Here's how the part is built. I have some questions about the finished solid (model axes, mm). Face numbers are marked on the shaded views. Coordinates: 2 decimals unless noted, no trailing zeros. Loops run counter-clockwise (first coordinate to the right, second up) from the corner with the lowest first, then second, coordinate; pieces in that order, holes last. Notation, with made-up numbers: (8, -37) -> (21, -37) arc R14 ccw to (21, -28) -> close; hole circle Ø1 at (85, 22). An arc over 180 degrees is marked (long way). Answer as a JSON object with one key per item and string values. Group by question number.
1) I want a section at C-C (x = 80). Write out the boundary of the cut face in (y, z), then the cut area to 3 significant figures.
2) I need wall thicknesses on probe 1 along Y at (x, z) = (80, -1); probe 2 along Y at (x, z) = (130, 3); probe 3 along X at (y, z) = (54, 11.25). Which ranges of each line are inside material? Lowest first, please. Write a range as [from, to].
3) I want a section at B-B (y = 50). Write out the boundary of the cut face in (x, z).
4) I'm going to push flat-ended pins straight in: pin 1 (10 mm diameter, centred on x = 72, z = 8.5, fed in from +Y); pin 2 (6 mm diameter, centred on x = 96.5, z = 9.5, fed in from +Y); pin 3 (12 mm diameter, centred on x = 54.5, z = 9.5, fed in from +Y). Where does each tip first touch, or does it pass through?
5) I want a section at A-A (z = 9.5). Write out the boundary of the cut face in (x, y).
6) I want a section at D-D (x = 30). Write out the boundary of the cut face in (y, z).
7) If we mould it in two halves opening along Y, with no side actions, what happens to the marked faces 1, 2 and 3? For each: +Y half, -Y half, draft (parallel to the pull), parting line (faces both ways), or undercut.
```python
from build123d import *

# Parameters (mm, degrees)
SKETCH1_R           = 20
SKETCH1_R_2         = 10
BOSS_EXTRUDE1_DEPTH = 12.5


with BuildPart() as part:
    # Sketch1 → Boss-Extrude1 (new, symmetric)
    with BuildSketch(Plane.XY):
        with BuildLine():
            Line((134.5, 64.309088021), (89, 78.618176043))
            ThreePointArc((89, 78.618176043), (80, 80), (71, 78.618176043))
            Line((71, 78.618176043), (25.5, 64.309088021))
            ThreePointArc((25.5, 64.309088021), (15, 50), (25.5, 35.690911979))
            Line((25.5, 35.690911979), (71, 21.381823957))
            ThreePointArc((71, 21.381823957), (80, 20), (89, 21.381823957))
            Line((89, 21.381823957), (134.5, 35.690911979))
            ThreePointArc((134.5, 35.690911979), (145, 50), (134.5, 64.309088021))
        make_face()
        with Locations((80, 50)):
            Circle(SKETCH1_R, mode=Mode.SUBTRACT)
        with Locations((130, 50)):
            Circle(SKETCH1_R_2, mode=Mode.SUBTRACT)
        with Locations(Location((30, 50, 0), (0, 0, 180))):
            Circle(SKETCH1_R_2, mode=Mode.SUBTRACT)
    extrude(amount=BOSS_EXTRUDE1_DEPTH, both=True)


solid = part.part
```
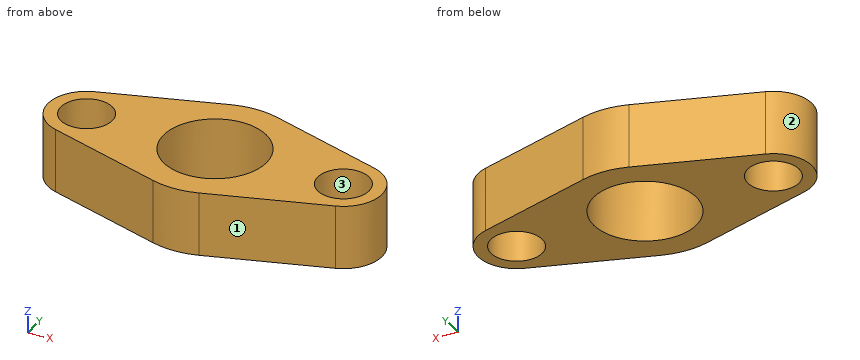
Determined:
{
 "1": {"outline": "(20, -12.5) -> (30, -12.5) -> (30, 12.5) -> (20, 12.5) -> close; (70, -12.5) -> (80, -12.5) -> (80, 12.5) -> (70, 12.5) -> close", "area": "500 mm^2"},
 "2": {"probe 1": "[20, 30], [70, 80]", "probe 2": "[34.28, 40], [60, 65.72]", "probe 3": "[15.54, 20.83], [39.17, 60.4], [99.6, 120.83], [139.17, 144.46]"},
 "3": {"outline": "(15, -12.5) -> (20, -12.5) -> (20, 12.5) -> (15, 12.5) -> close; (40, -12.5) -> (60, -12.5) -> (60, 12.5) -> (40, 12.5) -> close; (100, -12.5) -> (120, -12.5) -> (120, 12.5) -> (100, 12.5) -> close; (140, -12.5) -> (145, -12.5) -> (145, 12.5) -> (140, 12.5) -> close"},
 "4": {"pin 1": "y = 79.85", "pin 2": "y = 77.2", "pin 3": "y = 75.32"},
 "5": {"outline": "(25.5, 35.69) -> (71, 21.38) arc R30 ccw to (89, 21.38) -> (134.5, 35.69) arc R15 ccw to (134.5, 64.31) -> (89, 78.62) arc R30 ccw to (71, 78.62) -> (25.5, 64.31) arc R15 ccw to start; hole circle Ø20 at (30, 50); hole circle Ø40 at (80, 50); hole circle Ø20 at (130, 50)"},
 "6": {"outline": "(34.28, -12.5) -> (40, -12.5) -> (40, 12.5) -> (34.28, 12.5) -> close; (60, -12.5) -> (65.72, -12.5) -> (65.72, 12.5) -> (60, 12.5) -> close"},
 "7": {"face 1": "-Y half", "face 2": "parting line", "face 3": "undercut"}
}
